Design review of the part shown in the three views and the two pictorial views. Dimensions are in mm from the part's minimum x, y and z. A direction names the side the tool comes from. Round coordinates to 2 decimals unless told otherwise and drop trailing zeros. Write each loop counter-clockwise with the first axis right and the second up, starting at its lowest first coordinate (ties: lowest second). Pieces come first, ordered by that corner, then holes. Notation, with made-up numbers: (70.5, -18.5) - (102.5, -18.5) arc R9 ccw to (102.5, -3.5) - close; hole circle Ø4 at (36.5, 19). An arc over 180 degrees is marked (long way). Use one line per item in the form item = value.
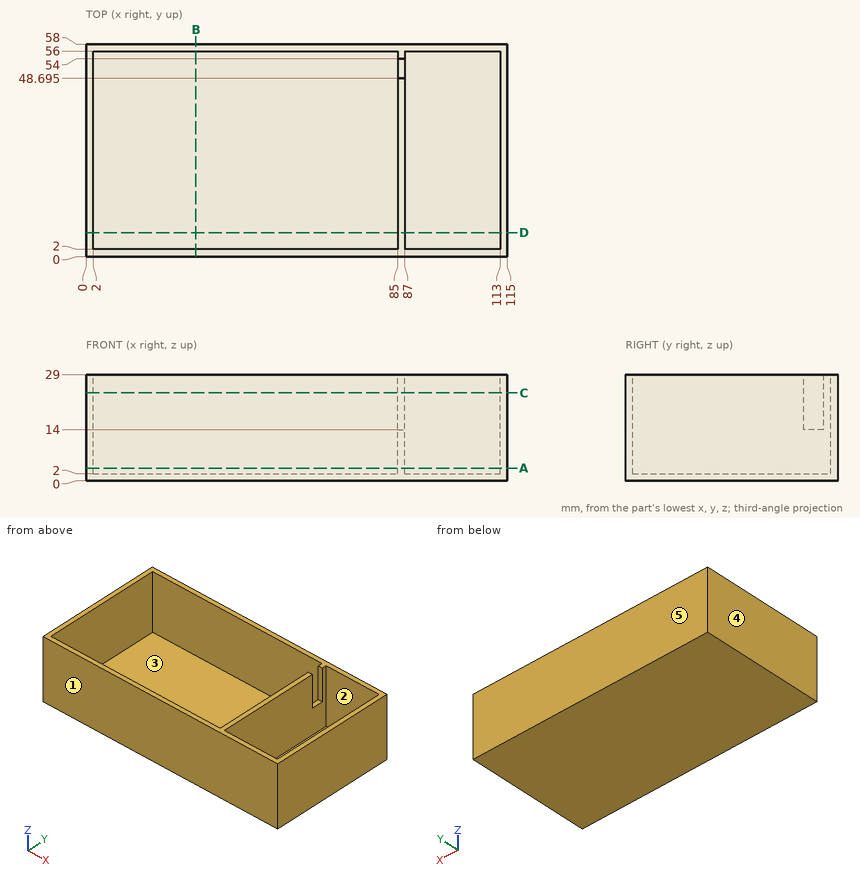
(1) Add section C-C on z = 24. Write out the cut boundary in (x, y) (1 decimal).
Geometry results:
outline = (0, 0) - (115, 0) - (115, 58) - (0, 58) - close; hole (2, 2) - (85, 2) - (85, 48.7) - (87, 48.7) - (87, 2) - (113, 2) - (113, 56) - (87, 56) - (87, 54) - (85, 54) - (85, 56) - (2, 56) - close
(2) Add section A-A on z = 3.5. Write out the cut boundary in (x, y).
Geometry results:
outline = (0, 0) - (115, 0) - (115, 58) - (0, 58) - close; hole (2, 2) - (85, 2) - (85, 56) - (2, 56) - close; hole (87, 2) - (113, 2) - (113, 56) - (87, 56) - close
(3) Add section D-D on y = 6.5. Write out the cut boundary in (x, z).
Geometry results:
outline = (0, 0) - (115, 0) - (115, 29) - (113, 29) - (113, 2) - (87, 2) - (87, 29) - (85, 29) - (85, 2) - (2, 2) - (2, 29) - (0, 29) - close
(4) To check wall thickness, follow L1, parallel to X at y = 18.5, z = 24.25; L2, parallel to Y at x = 39, z = 5.75; L3, parallel to X at y = 49, z = 20.5. State the ranges of each line that lie inside material, in increasing order.
Geometry results:
L1 = 0 to 2, 85 to 87, 113 to 115
L2 = 0 to 2, 56 to 58
L3 = 0 to 2, 113 to 115
(5) The part is to be moulded in two halves that separate along Y. For the marked faces 3, 4 and 5, say which applies: +Y half, -Y half, draft (parallel to the pull), parting line (faces both ways), or undercut.
Geometry results:
face_3 = undercut
face_4 = draft
face_5 = +Y half
(6) Insertion check: P1, Ø13, axis at x = 104, y = 38, coming from the +Z side; P2, Ø2, axis at x = 86, y = 52, coming from the +Z side. Each pin has a flat end and moves straight along its axis. Give the tip position at first contact, or say it passes through.
Geometry results:
P1 = 2
P2 = 14
(7) Add section B-B on x = 30. Write out the cut boundary in (y, z).
Geometry results:
outline = (0, 0) - (58, 0) - (58, 29) - (56, 29) - (56, 2) - (2, 2) - (2, 29) - (0, 29) - close
(8) Machinability: for the marked faces 1 and 2, which of the approach directions +Z, -Z, +X, -X, +Y, -Y give a long, thin tool a straight path to every point of the face, cutting with its end or side? Answer none if there is none.
Geometry results:
face_1 = +Z, -Z, +X, -X, -Y
face_2 = +Z
